Can you work these out from the model? Positions are in its coordinate system, mm. A direction names the side the tool comes from. Coordinates: 2 decimals unless noted, no trailing zeros. Order: outer loops, then holes, each group sorted by start corner. A loop starts at its lowest first (then second) coordinate and runs counter-clockwise, first axis right, second up. Notation, with made-up numbers: (-0.75, -14) -> (22.25, -14) arc R7 ccw to (22.25, -8) -> close; hole circle Ø9 at (26.25, -32). An arc over 180 degrees is marked (long way). Use a Markdown table: item, result. Add a question column.
1. For faces 4 (the cylindrical face through (-46.03, 47.39, -1.99)), 5 (the flat face through (-1, 81, 1)), 6 (the cylindrical face through (-0.85, 96.996, -0.014)), which set-ups out of +Z, -Z, +X, -X, +Y, -Y let a thin tool reach every point of the face, with its end or its side?
2. For pin 1 Ø1 at (y, z) = (5, 0.5) entering from +X; pin 2 Ø1 at (x, z) = (38, -2) entering from -Y; pin 3 Ø3 at (x, y) = (1, 0.5) entering from -Z; pin 4 Ø8 at (x, y) = (36, 101.5) entering from -Z, each with a flat end and sliding along its axis, tell me the tip position at first contact or that it passes through.
3. Suppose I cut it at A-A, the plane y = 0. List the corners of the cut face in (x, z) for me, then the cut area to 3 significant figures.
4. If I drill on line 1 along X through (y, z) = (46.5, 0.55); line 2 along Z through (x, y) = (10.5, 61.5); line 3 along Y through (x, z) = (-67, -1.55), over which ranges is the centre line in solid material (lowest first)? Write a range as from..to.
5. We'd pull the mould along X, two halves only. Please class faces 1 (the flat face through (0.2, 59.4, -3)), 2 (the cylindrical face through (-0.692, 70.797, -1.986)), 3 (the cylindrical face through (-60.174, 64.246, -1.986)): pulls with the +X half, pulls with the -X half, needs draft (parallel to the pull), parting line crosses it, or undercut.
6. Suppose I cut it at B-B, the plane z = -2.05. State how many separate pieces and enclosed holes the cut face has, then the cut area to 3 significant figures.
```python
from build123d import *

# Parameters (mm, degrees)
BOSS_EXTRUDE1_DEPTH      = 1
BOSS_EXTRUDE1_DEPTH_BACK = 1
SKETCH2_R                = 6.8
SKETCH2_R_2              = 4.8
BOSS_EXTRUDE2_DEPTH      = 2


with BuildPart() as part:
    # Sketch1 → Boss-Extrude1 (new, two sides: drawn at the far end of the back side and taken through both)
    with BuildSketch(Plane.XY.offset(-BOSS_EXTRUDE1_DEPTH_BACK)):
        with BuildLine():
            Line((-79.062875991, 94.223466504), (-76.491725553, 91.159288731))
            ThreePointArc((-76.491725553, 91.159288731), (-77.601037054, 78.479800256), (-64.921548578, 77.370488755))
            Line((-64.921548578, 77.370488755), (-62.35039814, 74.306310983))
            ThreePointArc((-62.35039814, 74.306310983), (-63.45970964, 61.626822507), (-50.780221165, 60.517511006))
            Line((-50.780221165, 60.517511006), (-48.209070726, 57.453333234))
            ThreePointArc((-48.209070726, 57.453333234), (-49.318382227, 44.773844759), (-36.638893752, 43.664533258))
            Line((-36.638893752, 43.664533258), (-34.067743313, 40.600355485))
            ThreePointArc((-34.067743313, 40.600355485), (-35.177054814, 27.92086701), (-22.497566339, 26.811555509))
            Line((-22.497566339, 26.811555509), (-19.9264159, 23.747377737))
            ThreePointArc((-19.9264159, 23.747377737), (-21.035727401, 11.067889261), (-8.356238926, 9.958577761))
            Line((-8.356238926, 9.958577761), (-5.785088487, 6.894399988))
            ThreePointArc((-5.785088487, 6.894399988), (-8.968372241, 0.753856314), (-6.854827722, -5.831923945))
            add(Edge.make_bspline(
                [(-6.854827722, -5.831923945), (-17.598880273, -8.504870382), (-21.273035539, -16.800000012)],
                knots=[1.880376726, 1.880376726, 1.880376726, 2.809825541, 2.809825541, 2.809825541], degree=2, weights=[1, 0.893945114, 1]))
            Line((-21.273035539, -16.800000012), (-15.574646072, -16.800000012))
            add(Edge.make_bspline(
                [(15.574646072, -16.800000012), (0, 4.91228076), (-15.574646072, -16.800000012)],
                knots=[3.615088165, 3.615088165, 3.615088165, 5.809689796, 5.809689796, 5.809689796], degree=2, weights=[1, 0.455999999, 1]))
            Line((15.574646072, -16.800000012), (21.273035539, -16.800000012))
            add(Edge.make_bspline(
                [(21.273035539, -16.800000012), (17.598880273, -8.504870382), (6.854827722, -5.831923945)],
                knots=[0.331767113, 0.331767113, 0.331767113, 1.261215927, 1.261215927, 1.261215927], degree=2, weights=[1, 0.893945114, 1]))
            ThreePointArc((6.854827722, -5.831923945), (8.968372241, 0.753856314), (5.785088487, 6.894399988))
            Line((5.785088487, 6.894399988), (8.356238926, 9.958577761))
            ThreePointArc((8.356238926, 9.958577761), (21.035727401, 11.067889261), (19.9264159, 23.747377737))
            Line((19.9264159, 23.747377737), (22.497566339, 26.811555509))
            ThreePointArc((22.497566339, 26.811555509), (35.177054814, 27.92086701), (34.067743313, 40.600355485))
            Line((34.067743313, 40.600355485), (36.638893752, 43.664533258))
            ThreePointArc((36.638893752, 43.664533258), (49.318382227, 44.773844759), (48.209070726, 57.453333234))
            Line((48.209070726, 57.453333234), (50.780221165, 60.517511006))
            ThreePointArc((50.780221165, 60.517511006), (63.45970964, 61.626822507), (62.35039814, 74.306310983))
            Line((62.35039814, 74.306310983), (64.921548578, 77.370488755))
            ThreePointArc((64.921548578, 77.370488755), (77.601037054, 78.479800256), (76.491725553, 91.159288731))
            Line((76.491725553, 91.159288731), (79.062875991, 94.223466504))
            ThreePointArc((79.062875991, 94.223466504), (91.742364467, 95.332778005), (90.633052966, 108.01226648))
            ThreePointArc((90.633052966, 108.01226648), (0, 141), (-90.633052966, 108.01226648))
            ThreePointArc((-90.633052966, 108.01226648), (-91.742364467, 95.332778005), (-79.062875991, 94.223466504))
        make_face()
        with BuildLine():
            Line((-73.572426121, 98.570269933), (-70.996961147, 95.500950298))
            ThreePointArc((-70.996961147, 95.500950298), (0, 119), (70.996961147, 95.500950298))
            Line((70.996961147, 95.500950298), (73.572426121, 98.570269933))
            ThreePointArc((73.572426121, 98.570269933), (0, 123), (-73.572426121, 98.570269933))
        make_face(mode=Mode.SUBTRACT)
        with BuildLine():
            Line((-59.403126055, 81.683955676), (-56.825521539, 78.612086233))
            ThreePointArc((-56.825521539, 78.612086233), (0, 97), (56.825521539, 78.612086233))
            Line((56.825521539, 78.612086233), (59.403126055, 81.683955676))
            ThreePointArc((59.403126055, 81.683955676), (0, 101), (-59.403126055, 81.683955676))
        make_face(mode=Mode.SUBTRACT)
        with BuildLine():
            Line((-45.218171715, 64.778985379), (-42.636323052, 61.702057961))
            ThreePointArc((-42.636323052, 61.702057961), (0, 75), (42.636323052, 61.702057961))
            Line((42.636323052, 61.702057961), (45.218171715, 64.778985379))
            ThreePointArc((45.218171715, 64.778985379), (0, 79), (-45.218171715, 64.778985379))
        make_face(mode=Mode.SUBTRACT)
        with BuildLine():
            Line((-30.999247112, 47.833530901), (-28.406987304, 44.744195962))
            ThreePointArc((-28.406987304, 44.744195962), (0, 53), (28.406987304, 44.744195962))
            Line((28.406987304, 44.744195962), (30.999247112, 47.833530901))
            ThreePointArc((30.999247112, 47.833530901), (0, 57), (-30.999247112, 47.833530901))
        make_face(mode=Mode.SUBTRACT)
        with BuildLine():
            Line((-16.680712092, 30.769365351), (-14.049449019, 27.63354813))
            ThreePointArc((-14.049449019, 27.63354813), (0, 31), (14.049449019, 27.63354813))
            Line((14.049449019, 27.63354813), (16.680712092, 30.769365351))
            ThreePointArc((16.680712092, 30.769365351), (0, 35), (-16.680712092, 30.769365351))
        make_face(mode=Mode.SUBTRACT)
        with BuildLine():
            Line((-1.679074368, 12.891109699), (0, 10.890066788))
            Line((0, 10.890066788), (1.679074368, 12.891109699))
            ThreePointArc((1.679074368, 12.891109699), (0, 13), (-1.679074368, 12.891109699))
        make_face(mode=Mode.SUBTRACT)
    extrude(amount=BOSS_EXTRUDE1_DEPTH + BOSS_EXTRUDE1_DEPTH_BACK)

    # Sketch2 → Boss-Extrude2 (add)
    # profile 1 of 7: a face of its own
    with BuildSketch(Plane(origin=(0, 0, -1), x_dir=(-1, 0, 0), z_dir=(0, 0, -1))):
        Circle(SKETCH2_R)
        Circle(SKETCH2_R_2, mode=Mode.SUBTRACT)
    # profile 2 of 7: a face of its own
    with BuildSketch(Plane(origin=(0, 0, -1), x_dir=(-1, 0, 0), z_dir=(0, 0, -1))):
        with BuildLine():
            ThreePointArc((80.477008733, 95.908764278), (0, 125.2), (-80.477008733, 95.908764278))
            ThreePointArc((-80.477008733, 95.908764278), (-90.057066692, 96.746910746), (-89.218920224, 106.326968705))
            ThreePointArc((-89.218920224, 106.326968705), (0, 138.8), (89.218920224, 106.326968705))
            ThreePointArc((89.218920224, 106.326968705), (90.057066692, 96.746910746), (80.477008733, 95.908764278))
        make_face()
        with BuildLine():
            ThreePointArc((81.762583952, 97.440853165), (0, 127.2), (-81.762583952, 97.440853165))
            ThreePointArc((-81.762583952, 97.440853165), (-88.524977806, 98.032485965), (-87.933345005, 104.794879819))
            ThreePointArc((-87.933345005, 104.794879819), (0, 136.8), (87.933345005, 104.794879819))
            ThreePointArc((87.933345005, 104.794879819), (88.524977806, 98.032485965), (81.762583952, 97.440853165))
        make_face(mode=Mode.SUBTRACT)
    # profile 3 of 7: a face of its own
    with BuildSketch(Plane(origin=(0, 0, -1), x_dir=(-1, 0, 0), z_dir=(0, 0, -1))):
        with BuildLine():
            ThreePointArc((75.077592811, 89.473990956), (0, 116.8), (-75.077592811, 89.473990956))
            ThreePointArc((-75.077592811, 89.473990956), (-75.915739279, 79.893932997), (-66.33568132, 79.05578653))
            ThreePointArc((-66.33568132, 79.05578653), (0, 103.2), (66.33568132, 79.05578653))
            ThreePointArc((66.33568132, 79.05578653), (75.915739279, 79.893932997), (75.077592811, 89.473990956))
        make_face()
        with BuildLine():
            ThreePointArc((73.792017592, 87.94190207), (0, 114.8), (-73.792017592, 87.94190207))
            ThreePointArc((-73.792017592, 87.94190207), (-74.383650392, 81.179508217), (-67.621256539, 80.587875416))
            ThreePointArc((-67.621256539, 80.587875416), (0, 105.2), (67.621256539, 80.587875416))
            ThreePointArc((67.621256539, 80.587875416), (74.383650392, 81.179508217), (73.792017592, 87.94190207))
        make_face(mode=Mode.SUBTRACT)
    # profile 4 of 7: a face of its own
    with BuildSketch(Plane(origin=(0, 0, -1), x_dir=(-1, 0, 0), z_dir=(0, 0, -1))):
        with BuildLine():
            ThreePointArc((23.91169908, 28.496853284), (33.491757039, 29.334999751), (32.653610572, 38.91505771))
            ThreePointArc((32.653610572, 38.91505771), (0, 50.8), (-32.653610572, 38.91505771))
            ThreePointArc((-32.653610572, 38.91505771), (-33.491757039, 29.334999751), (-23.91169908, 28.496853284))
            ThreePointArc((-23.91169908, 28.496853284), (0, 37.2), (23.91169908, 28.496853284))
        make_face()
        with BuildLine():
            ThreePointArc((25.1972743, 30.02894217), (31.959668153, 30.620574971), (31.368035353, 37.382968824))
            ThreePointArc((31.368035353, 37.382968824), (0, 48.8), (-31.368035353, 37.382968824))
            ThreePointArc((-31.368035353, 37.382968824), (-31.959668153, 30.620574971), (-25.1972743, 30.02894217))
            ThreePointArc((-25.1972743, 30.02894217), (0, 39.2), (25.1972743, 30.02894217))
        make_face(mode=Mode.SUBTRACT)
    # profile 5 of 7: a face of its own
    with BuildSketch(Plane(origin=(0, 0, -1), x_dir=(-1, 0, 0), z_dir=(0, 0, -1))):
        with BuildLine():
            ThreePointArc((38.053026493, 45.349831033), (47.633084453, 46.1879775), (46.794937985, 55.768035459))
            ThreePointArc((46.794937985, 55.768035459), (0, 72.8), (-46.794937985, 55.768035459))
            ThreePointArc((-46.794937985, 55.768035459), (-47.633084453, 46.1879775), (-38.053026493, 45.349831033))
            ThreePointArc((-38.053026493, 45.349831033), (0, 59.2), (38.053026493, 45.349831033))
        make_face()
        with BuildLine():
            ThreePointArc((39.338601713, 46.881919919), (46.100995566, 47.473552719), (45.509362766, 54.235946573))
            ThreePointArc((45.509362766, 54.235946573), (0, 70.8), (-45.509362766, 54.235946573))
            ThreePointArc((-45.509362766, 54.235946573), (-46.100995566, 47.473552719), (-39.338601713, 46.881919919))
            ThreePointArc((-39.338601713, 46.881919919), (0, 61.2), (39.338601713, 46.881919919))
        make_face(mode=Mode.SUBTRACT)
    # profile 6 of 7: a face of its own
    with BuildSketch(Plane(origin=(0, 0, -1), x_dir=(-1, 0, 0), z_dir=(0, 0, -1))):
        with BuildLine():
            ThreePointArc((52.194353907, 62.202808781), (61.774411866, 63.040955249), (60.936265398, 72.621013208))
            ThreePointArc((60.936265398, 72.621013208), (0, 94.8), (-60.936265398, 72.621013208))
            ThreePointArc((-60.936265398, 72.621013208), (-61.774411866, 63.040955249), (-52.194353907, 62.202808781))
            ThreePointArc((-52.194353907, 62.202808781), (0, 81.2), (52.194353907, 62.202808781))
        make_face()
        with BuildLine():
            ThreePointArc((53.479929126, 63.734897667), (60.242322979, 64.326530468), (59.650690179, 71.088924321))
            ThreePointArc((59.650690179, 71.088924321), (0, 92.8), (-59.650690179, 71.088924321))
            ThreePointArc((-59.650690179, 71.088924321), (-60.242322979, 64.326530468), (-53.479929126, 63.734897667))
            ThreePointArc((-53.479929126, 63.734897667), (0, 83.2), (53.479929126, 63.734897667))
        make_face(mode=Mode.SUBTRACT)
    # profile 7 of 7: a face of its own
    with BuildSketch(Plane(origin=(0, 0, -1), x_dir=(-1, 0, 0), z_dir=(0, 0, -1))):
        with BuildLine():
            ThreePointArc((-18.512283159, 22.062079962), (-19.350429626, 12.482022003), (-9.770371667, 11.643875535))
            ThreePointArc((-9.770371667, 11.643875535), (0, 15.2), (9.770371667, 11.643875535))
            ThreePointArc((9.770371667, 11.643875535), (19.350429626, 12.482022003), (18.512283159, 22.062079962))
            ThreePointArc((18.512283159, 22.062079962), (0, 28.8), (-18.512283159, 22.062079962))
        make_face()
        with BuildLine():
            ThreePointArc((-17.22670794, 20.529991076), (-17.81834074, 13.767597222), (-11.055946887, 13.175964422))
            ThreePointArc((-11.055946887, 13.175964422), (0, 17.2), (11.055946887, 13.175964422))
            ThreePointArc((11.055946887, 13.175964422), (17.81834074, 13.767597222), (17.22670794, 20.529991076))
            ThreePointArc((17.22670794, 20.529991076), (0, 26.8), (-17.22670794, 20.529991076))
        make_face(mode=Mode.SUBTRACT)
    extrude(amount=BOSS_EXTRUDE2_DEPTH)


solid = part.part
```
Worked out:
| question | item | result |
|---|---|---|
| 1 | face 4 | -Z |
| 1 | face 5 | +Z, +X, -X, +Y, -Y |
| 1 | face 6 | +Z, -Z |
| 2 | pin 1 | stops at x = 7.79 |
| 2 | pin 2 | stops at y = 45.01 |
| 2 | pin 3 | stops at z = -1 |
| 2 | pin 4 | stops at z = -3 |
| 3 | outline | (-9, -1) -> (-6.8, -1) -> (-6.8, -3) -> (-4.8, -3) -> (-4.8, -1) -> (4.8, -1) -> (4.8, -3) -> (6.8, -3) -> (6.8, -1) -> (9, -1) -> (9, 1) -> (-9, 1) -> close |
| 3 | area | 44.0 mm² |
| 4 | line 1 | x = -50.46..-29.88, -25.43..25.43, 29.88..50.46 |
| 4 | line 2 | z = -1..1 |
| 4 | line 3 | y = 78.56..81.11, 93.22..95.67, 105.76..108.12, 119.27..121.56 |
| 5 | face 1 | needs draft |
| 5 | face 2 | undercut |
| 5 | face 3 | undercut |
| 6 | separate pieces | 7 |
| 6 | enclosed holes | 7 |
| 6 | area | 3,090 mm² |
